Can you work these out from the drawing? Everything is in mm from the part's minimum corner. Round coordinates to 2 decimals unless told otherwise and drop trailing zeros. Loops run counter-clockwise (first coordinate to the right, second up) from the corner with the lowest first, then second, coordinate; pieces in that order, holes last. Notation, with made-up numbers: M -28,27.5 L -22,27.5 A12 ccw -22,33.5 Z; hole C -6.75,-33 d3. An arc over 180 degrees is marked long. Return JSON: item names as keys, results as strings. Group by question number.
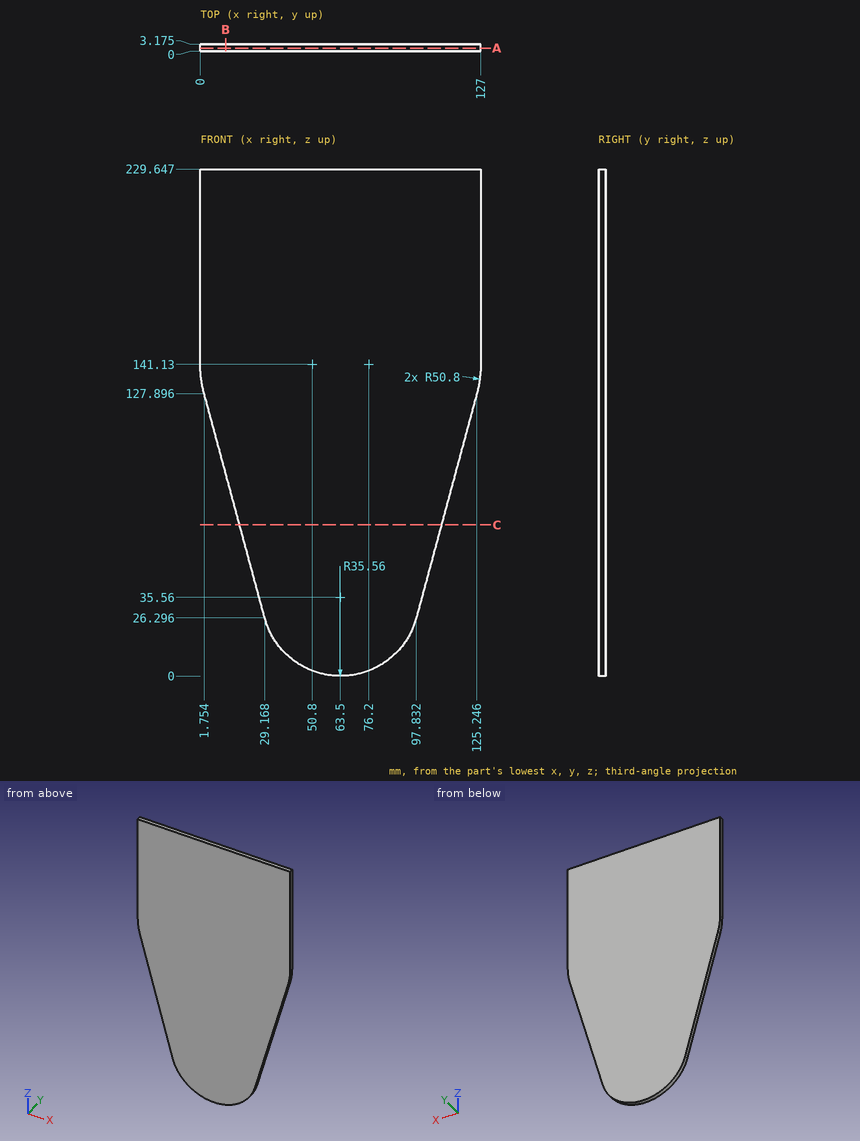
1. I need wall thicknesses on probe 1 along X at (y, z) = (1.2, 68) (1 decimal); probe 2 along X at (y, z) = (1.9, 101); probe 3 along Z at (x, y) = (72.5, 2.8). Which ranges of each line are inside material? Lowest first, please.
2. If we section it at A-A, the plane y = 1.3: Please give me the cut outline in (x, z), then the cut area to 3 significant figures.
3. If we section it at B-B, the plane x = 11.5: Please give me the cut outline in (y, z) (1 decimal).
4. If we section it at C-C, the plane z = 68.5: Please give me the cut outline in (x, y) (1 decimal).
5. I'm going to push a flat-ended pin straight in: pin 1 Ø1.5 at (y, z) = (2.5, 81.5) entering from -X. Where does the tip first touch, or does it pass through?
Geometry results:
{
 "1": {"probe 1": "17.9 to 109.1", "probe 2": "9.01 to 117.99", "probe 3": "1.16 to 229.65"},
 "2": {"outline": "M 0,141.13 A50.8 ccw 1.75,127.9 L 29.17,26.3 A35.56 ccw 97.83,26.3 L 125.25,127.9 A50.8 ccw 127,141.13 L 127,229.65 L 0,229.65 Z", "area": "24,000 mm^2"},
 "3": {"outline": "M 0,91.8 L 3.2,91.8 L 3.2,229.6 L 0,229.6 Z"},
 "4": {"outline": "M 17.8,0 L 109.2,0 L 109.2,3.2 L 17.8,3.2 Z"},
 "5": {"pin 1": "x = 14.07"}
}
